Geometry check sheet. Reference: the model listing, model coordinates, mm. A direction names the side the tool comes from. Give positions to 0.01 mm unless a question says otherwise; leave off trailing zeros. Order: outer loops, then holes, each group sorted by start corner. A loop starts at its lowest first (then second) coordinate and runs counter-clockwise, first axis right, second up. Notation, with made-up numbers: M -31,10 L 27,10 A17 ccw 27,18 Z; hole C 71.25,-16 d11. An arc over 180 degrees is marked long. Answer as CSV lines item,"result". Start each with the question number.
Q1. Thickness scan on line 1 (Z direction, x = 393, y = 122); line 2 (Y direction, x = 220, z = -27) (3 decimals); line 3 (Z direction, x = 209, y = 85) (3 decimals). Record the ranges inside material, lowest first.
Q2. Go/stop test with flat-tipped pins: pin 1 (5 mm diameter, centred on x = 530, z = -43.5, fed in from -Y); pin 2 (1.5 mm diameter, centred on x = 154, y = 116, fed in from +Z) (3 decimals). Record where each tip stops, or that it passes through.
Q3. Mould release check, pull along Z, two halves, no side actions. Record for faces 1 (the flat face through (322, 89, -152.4)), 2 (the cylindrical face through (397.38, 122.26, -48.89)), 3 (the cylindrical face through (226.56, 122.26, -25.8)), 4 (the flat face through (322, 120.65, -72)): +Z half, -Z half, draft (parallel to the pull), parting line (faces both ways), or undercut.
Q4. Section check D-D, the plane y = 89.5. Record the boundary of the cut face in (x, z) (3 decimals).
Q5. Section check C-C, the plane z = -97. Record the boundary of the cut face in (x, y) (3 decimals).
Q6. Section check A-A, the plane z = -51.5. Record the boundary of the cut face in (x, y) (3 decimals).
Q7. Set-up check for faces 5 (the flat face through (322, 123.825, -74)), 6 (the flat face through (322, 90, -149.225)): record each of +Z, -Z, +X, -X, +Y, -Y from which the full face is reachable in a straight line by a thin tool's end or side.
```python
from build123d import *

# Parameters (mm, degrees)
BASE_FLANGE1_DEPTH = 654.05
SKETCH6_R          = 21.9075
CUT_EXTRUDE1_DEPTH = 3.175
SKETCH7_R          = 2.4257
CUT_EXTRUDE2_DEPTH = 683.89076222
SKETCH8_R          = 2.4257
CUT_EXTRUDE3_DEPTH = 683.89076222
SKETCH9_R          = 2.4257
CUT_EXTRUDE4_DEPTH = 683.89076222
FILLET1_R          = 3.175
SKETCH10_W         = 152.4
SKETCH10_H         = 61.9125
CUT_EXTRUDE5_DEPTH = 683.89076222
FILLET2_R          = 3.175


# Sheet-metal steps are written as plain solids
with BuildPart() as part:
    # Sketch1 → Base-Flange1 (new body)
    with BuildSketch(Plane(origin=(0, 0, 0), x_dir=(0, 0, -1), z_dir=(1, 0, 0))):
        with BuildLine():
            Line((0, 0), (146.05, 0))
            ThreePointArc((146.05, 0), (150.540128061, 1.859871939), (152.4, 6.35))
            Line((152.4, 6.35), (152.4, 117.475))
            ThreePointArc((152.4, 117.475), (150.540128061, 121.965128061), (146.05, 123.825))
            Line((146.05, 123.825), (0, 123.825))
            Line((0, 123.825), (0, 120.65))
            Line((0, 120.65), (146.05, 120.65))
            ThreePointArc((146.05, 120.65), (148.29506403, 119.72006403), (149.225, 117.475))
            Line((149.225, 117.475), (149.225, 6.35))
            ThreePointArc((149.225, 6.35), (148.29506403, 4.10493597), (146.05, 3.175))
            Line((146.05, 3.175), (0, 3.175))
            Line((0, 3.175), (0, 0))
        make_face()
    extrude(amount=BASE_FLANGE1_DEPTH)

    # Sketch6 → Cut-Extrude1 (cut)
    with BuildSketch(Plane(origin=(0, 123.825, 0), x_dir=(1, 0, 0), z_dir=(0, 1, 0))):
        with Locations(Location((234.95, 46.0375, 0), (0, 0, 270))):
            Circle(SKETCH6_R)
    cut_extrude1 = extrude(amount=-CUT_EXTRUDE1_DEPTH, mode=Mode.SUBTRACT)

    # Sketch7 → Cut-Extrude2 (cut, through all)
    with BuildSketch(Plane(origin=(0, 123.825, 0), x_dir=(1, 0, 0), z_dir=(0, 1, 0))):
        with Locations(Location((234.95, 12.2555, 0), (0, 0, 270))):
            Circle(SKETCH7_R)
        with Locations(Location((234.95, 79.8195, 0), (0, 0, 270))):
            Circle(SKETCH7_R)
        with Locations(Location((209.55, 12.2555, 0), (0, 0, 270))):
            Circle(SKETCH7_R)
        with Locations(Location((260.35, 12.2555, 0), (0, 0, 270))):
            Circle(SKETCH7_R)
        with Locations(Location((260.35, 79.8195, 0), (0, 0, 270))):
            Circle(SKETCH7_R)
        with Locations(Location((209.55, 79.8195, 0), (0, 0, 270))):
            Circle(SKETCH7_R)
    cut_extrude2 = extrude(amount=-CUT_EXTRUDE2_DEPTH, mode=Mode.SUBTRACT)

    # Sketch8 → Cut-Extrude3 (cut, through all)
    with BuildSketch(Plane(origin=(0, 123.825, 0), x_dir=(1, 0, 0), z_dir=(0, 1, 0))):
        with Locations(Location((644.525, 12.7, 0), (0, 0, 270))):
            Circle(SKETCH8_R)
        with Locations(Location((644.525, 71.4375, 0), (0, 0, 270))):
            Circle(SKETCH8_R)
        with Locations(Location((644.525, 130.175, 0), (0, 0, 270))):
            Circle(SKETCH8_R)
        with Locations(Location((9.525, 130.175, 0), (0, 0, 270))):
            Circle(SKETCH8_R)
        with Locations(Location((9.525, 71.4375, 0), (0, 0, 270))):
            Circle(SKETCH8_R)
        with Locations(Location((9.525, 12.7, 0), (0, 0, 270))):
            Circle(SKETCH8_R)
    extrude(amount=-CUT_EXTRUDE3_DEPTH, mode=Mode.SUBTRACT)

    # Sketch9 → Cut-Extrude4 (cut, through all)
    with BuildSketch(Plane(origin=(0, 0, -152.4), x_dir=(-1, 0, 0), z_dir=(0, 0, -1))):
        with Locations((-644.525, 74.6125)):
            Circle(SKETCH9_R)
        with Locations((-644.525, 49.2125)):
            Circle(SKETCH9_R)
        with Locations((-9.525, 49.2125)):
            Circle(SKETCH9_R)
        with Locations((-9.525, 74.6125)):
            Circle(SKETCH9_R)
        with Locations((-644.525, 100.0125)):
            Circle(SKETCH9_R)
        with Locations((-644.525, 23.8125)):
            Circle(SKETCH9_R)
        with Locations((-9.525, 23.8125)):
            Circle(SKETCH9_R)
        with Locations((-9.525, 100.0125)):
            Circle(SKETCH9_R)
    extrude(amount=-CUT_EXTRUDE4_DEPTH, mode=Mode.SUBTRACT)

    # Fillet1
    fillet1_edges = [part.edges().sort_by_distance(p)[0] for p in [
        (0, 1.5875, 0),
        (0, 122.2375, 0),
        (654.05, 1.5875, 0),
        (654.05, 122.2375, 0),
    ]]
    fillet(fillet1_edges, radius=FILLET1_R)

    # Sketch10 → Cut-Extrude5 (cut, through all)
    with BuildSketch(Plane(origin=(654.05, 0, 0), x_dir=(0, 0, -1), z_dir=(1, 0, 0))):
        with Locations((76.2, 30.95625)):
            Rectangle(SKETCH10_W, SKETCH10_H)
    extrude(amount=-CUT_EXTRUDE5_DEPTH, mode=Mode.SUBTRACT)

    # Fillet2
    fillet2_edges = [part.edges().sort_by_distance(p)[0] for p in [
        (654.05, 61.9125, -150.8125),
        (0, 61.9125, -150.8125),
    ]]
    fillet(fillet2_edges, radius=FILLET2_R)

    # Mirror1: Cut-Extrude1, Cut-Extrude2 across plane
    add(cut_extrude1.mirror(Plane.ZY.offset(-327.025)), mode=Mode.SUBTRACT)
    add(cut_extrude2.mirror(Plane.ZY.offset(-327.025)), mode=Mode.SUBTRACT)


solid = part.part
```
Answer block:
1,line 1,"z = -150.5 to -82.14, -77.5 to -14.58, -9.93 to 0"
1,line 2,"y = 120.65 to 123.825"
1,line 3,"z = -152.4 to -149.225"
2,pin 1,"stops at y = 120.65"
2,pin 2,"stops at z = -149.225"
3,face 1,"-Z half"
3,face 2,"undercut"
3,face 3,"undercut"
3,face 4,"draft"
4,outline,"M 0,-152.4 L 654.05,-152.4 L 654.05,-149.225 L 0,-149.225 Z"
5,outline,"M 0,120.65 L 654.05,120.65 L 654.05,123.825 L 0,123.825 Z"
6,outline,"M 0,120.65 L 213.734,120.65 L 213.734,123.825 L 0,123.825 Z; M 256.166,120.65 L 397.884,120.65 L 397.884,123.825 L 256.166,123.825 Z; M 440.316,120.65 L 654.05,120.65 L 654.05,123.825 L 440.316,123.825 Z"
7,face 5,"+Z, -Z, +X, -X, +Y"
7,face 6,"+Z, +X, -X, -Y"
